```python
from build123d import *

# Parameters (mm, degrees)
F0_W      = 300
F0_H      = 200
F1_DEPTH  = 40
F2_R      = 20
F3_SIZE   = 5
F4_W      = 20
F4_H      = 10
F5_DEPTH  = 125
F6_W      = 10
F6_H      = 20
F7_DEPTH  = 200
F7_TAPER  = 0.5
F8_W      = 10
F8_H      = 10
F9_DEPTH  = 20
F10_R     = 3
F14_W     = 8
F14_H     = 8
F15_DEPTH = 5


with BuildPart() as f1:
    # F0 (on Top) → F1 (new body)
    with BuildSketch(Plane.XY):
        Rectangle(F0_W, F0_H)
    extrude(amount=F1_DEPTH)

    # F2
    f2_edges = [f1.edges().sort_by_distance(p)[0] for p in [
        (-150, -100, 20),
        (150, -100, 20),
        (150, 100, 20),
        (-150, 100, 20),
    ]]
    fillet(f2_edges, radius=F2_R)

    # F3
    f3_edges = [f1.edges().sort_by_distance(p)[0] for p in [
        (0, -100, 40),
        (0, -100, 0),
    ]]
    chamfer(f3_edges, length=F3_SIZE)

    # F4 (on Right) → F5 (join, symmetric)
    with BuildSketch(Plane.YZ):
        with Locations((100, 10)):
            Rectangle(F4_W, F4_H)
    extrude(amount=F5_DEPTH, both=True)

    # F6 (on face) → F7 (join)
    with BuildSketch(Plane.XY.offset(15)):
        with Locations((-120, 115)):
            Rectangle(F6_W, F6_H)
        with Locations((-40, 115)):
            Rectangle(F6_W, F6_H)
        with Locations((40, 115)):
            Rectangle(F6_W, F6_H)
        with Locations((120, 115)):
            Rectangle(F6_W, F6_H)
    extrude(amount=F7_DEPTH, taper=F7_TAPER)

    # F8 (on face) → F9 (join, symmetric)
    with BuildSketch(Plane(origin=(0, 110, 0), x_dir=(-1, 0, 0), z_dir=(0, 1, 0))):
        with Locations((0, 13)):
            Rectangle(F8_W, F8_H)
    extrude(amount=F9_DEPTH, both=True)

    # F13: sweep along a path in F12
    with BuildLine(Plane.XY.offset(13)) as f13_path:
        Line((0, 130), (0, 150))
        Line((0, 150), (0, 170))
        ThreePointArc((0, 170), (-5.8578643763, 184.1421356237), (-20, 190))
        Line((-20, 190), (-230, 190))
        ThreePointArc((-230, 190), (-244.1421356237, 184.1421356237), (-250, 170))
        Line((-250, 170), (-250, 90))
        ThreePointArc((-250, 90), (-255.8578643763, 75.8578643763), (-270, 70))
        Line((-270, 70), (-500, 70))
    # F10 (on face) → F13 (sweep)
    with BuildSketch(Plane(origin=(0, 130, 0), x_dir=(-1, 0, 0), z_dir=(0, 1, 0))):
        with Locations((0, 13)):
            Circle(F10_R)
    sweep(path=f13_path.line)

    # F14 (on face) → F15 (join)
    with BuildSketch(Plane(origin=(-500, 0, 0), x_dir=(0, -1, 0), z_dir=(-1, 0, 0))):
        with Locations((-70, 13)):
            Rectangle(F14_W, F14_H)
    extrude(amount=F15_DEPTH)


solid = f1.part
```
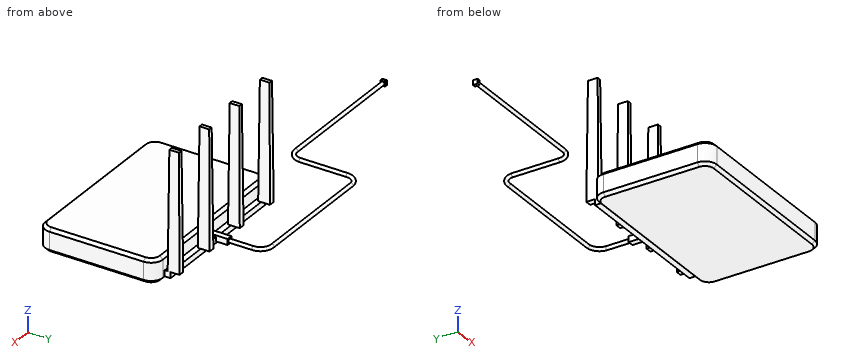
CAD build for the part. Positions are in the model's coordinates, mm. Coordinates: 2 decimals unless noted, no trailing zeros. Write each loop counter-clockwise with the first axis right and the second up, starting at its lowest first coordinate (ties: lowest second). Pieces come first, ordered by that corner, then holes.
(1) Cut at D-D, the plane x = 65. List the corners of the cut face in (y, z).
(2) Cut at C-C, the plane y = -16. List the corners of the cut face in (x, z).
(3) Cut at A-A, the plane x = -103. List the corners of the cut face in (y, z).
(4) Cut at B-B, the plane z = 112. List the corners of the cut face in (x, y).
(5) Flat gauge pins, fed straight in: pin 1 (3 mm diameter, centred on y = 105.5, z = 11.5, fed in from +X); pin 2 (5 mm diameter, centred on x = -31, y = 104.5, fed in from -Z); pin 3 (5 mm diameter, centred on x = 40.5, y = 116, fed in from -Z). Where does each tip first touch, or does it go through?
(6) Drill centre lines: probe 1 along Z at (x, y) = (-11, 73); probe 2 along X at (y, z) = (-28, 25); probe 3 along Y at (x, z) = (-41, 201). Where is each one in solid material? Low to high.
Geometry says:
1. outline: (-100, 5) - (-95, 0) - (95, 0) - (100, 5) - (110, 5) - (110, 15) - (100, 15) - (100, 35) - (95, 40) - (-95, 40) - (-100, 35) - close
2. outline: (-150, 5) - (-145, 0) - (145, 0) - (150, 5) - (150, 35) - (145, 40) - (-145, 40) - (-150, 35) - close
3. outline: (-100, 5) - (-95, 0) - (95, 0) - (100, 5) - (110, 5) - (110, 15) - (100, 15) - (100, 35) - (95, 40) - (-95, 40) - (-100, 35) - close; circle Ø6 at (190, 13)
4. outline: (-124.15, 105.85) - (-115.85, 105.85) - (-115.85, 124.15) - (-124.15, 124.15) - close; (-44.15, 105.85) - (-35.85, 105.85) - (-35.85, 124.15) - (-44.15, 124.15) - close; (35.85, 105.85) - (44.15, 105.85) - (44.15, 124.15) - (35.85, 124.15) - close; (115.85, 105.85) - (124.15, 105.85) - (124.15, 124.15) - (115.85, 124.15) - close
5. pin 1: stops at x = 125
5. pin 2: stops at z = 5
5. pin 3: stops at z = 15
6. probe 1: z = 0 to 40
6. probe 2: x = -150 to 150
6. probe 3: y = 106.62 to 123.38
